The model under review builds one solid part; all positions refer to its coordinate system, in mm. A direction names the side the tool comes from. Round coordinates to 2 decimals unless told otherwise and drop trailing zeros. Order: outer loops, then holes, each group sorted by start corner. A loop starts at its lowest first (then second) coordinate and runs counter-clockwise, first axis right, second up.
```python
from build123d import *

# Parameters (mm, degrees)
F0_W     = 32.5
F0_H     = 50.1
F2_DEPTH = 1.6
F3_START = 4.05
F1_W     = 16.8
F1_H     = 13.2
F3_DEPTH = 21


with BuildPart() as f2:
    # F0 (on Top) → F2 (new body)
    with BuildSketch(Plane.XY):
        Rectangle(F0_W, F0_H)
    extrude(amount=-F2_DEPTH)

    # F1 (on Front) → F3 (join)
    with BuildSketch(Plane.XZ.offset(F3_START)):
        with Locations((0, 6.6)):
            Rectangle(F1_W, F1_H)
    extrude(amount=F3_DEPTH)


solid = f2.part
```
(1) Draft analysis for pull direction Z (two halves, no side actions). For faces 6 (the flat face through (16.25, 0, -1)), 7 (the flat face through (0, 0, -1.6)), 8 (the flat face through (0, -14, 13.2)), state which applies: pulls with the +Z half, pulls with the -Z half, needs draft (parallel to the pull), parting line crosses it, or undercut.
Data:
face 6: needs draft
face 7: pulls with the -Z half
face 8: pulls with the +Z half
(2) Consider section C-C (z = 5). Write out the cut boundary in (x, y), and give its area (3 significant figures).
Data:
outline: (-8.4, -25.05) - (8.4, -25.05) - (8.4, -4.05) - (-8.4, -4.05) - close
area: 353 mm2
(3) Insertion check: pin 1 (12 mm diameter, centred on x = 10, y = 19, fed in from +Z); pin 2 (6.5 mm diameter, centred on y = -19, z = 8, fed in from +X); pin 3 (2 mm diameter, centred on y = -16, z = 3, fed in from -X). Each pin has a flat end and moves straight along its axis. Give the tip position at first contact, or say it passes through.
Data:
pin 1: stops at z = 0
pin 2: stops at x = 8.4
pin 3: stops at x = -8.4
(4) Consider section A-A (x = -1). Write out the cut boundary in (y, z), and give its area (3 significant figures).
Data:
outline: (-25.05, -1.6) - (25.05, -1.6) - (25.05, 0) - (-4.05, 0) - (-4.05, 13.2) - (-25.05, 13.2) - close
area: 357 mm2
(5) To check wall thickness, follow probe 1 along Z at (x, y) = (-9, -15.5); probe 2 along Y at (x, z) = (-6.5, 11.75); probe 3 along X at (y, z) = (-8.5, 10.25). State the ranges of each line that lie inside material, in increasing order.
Data:
probe 1: z = -1.6 to 0
probe 2: y = -25.05 to -4.05
probe 3: x = -8.4 to 8.4
(6) For faces 1 (the flat face through (0, -4.05, 7)), 2 (the flat face through (0, 25.05, -1)), 3 (the flat face through (-8.4, -14, 7)), 4 (the flat face through (8.4, -14, 7)), 5 (the flat face through (-16.25, 0, -1)), list the 3-axis set-ups (+Z, -Z, +X, -X, +Y, -Y) from which the entire face can be reached by the end or side of a thin tool; tool diameter is ignored.
Data:
face 1: +Z, +X, -X, +Y
face 2: +Z, -Z, +X, -X, +Y
face 3: +Z, -X, +Y, -Y
face 4: +Z, +X, +Y, -Y
face 5: +Z, -Z, -X, +Y, -Y
(7) Consider section B-B (y = 12). Write out the cut boundary in (x, z).
Data:
outline: (-16.25, -1.6) - (16.25, -1.6) - (16.25, 0) - (-16.25, 0) - close
